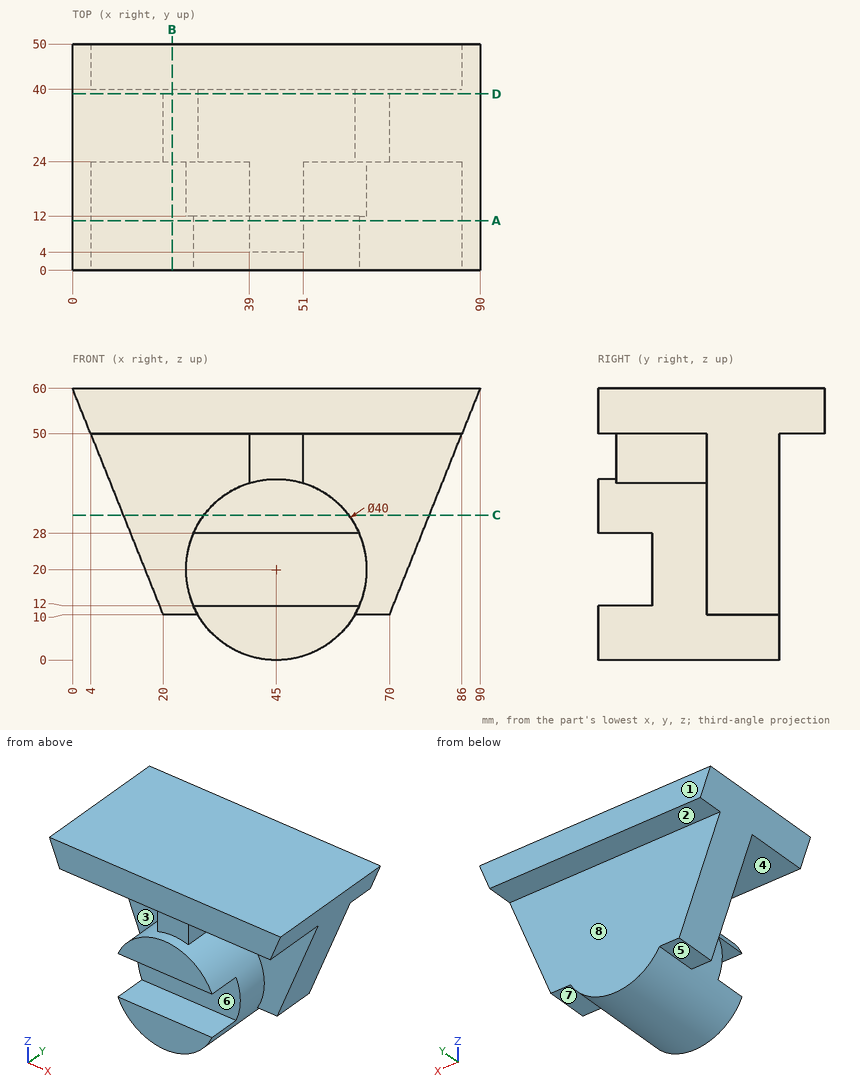
Design review of the part shown in the three views and the two pictorial views. Dimensions are in mm from the part's minimum x, y and z. A direction names the side the tool comes from. Give positions to 0.01 mm unless a question says otherwise; leave off trailing zeros. Write each loop counter-clockwise with the first axis right and the second up, starting at its lowest first coordinate (ties: lowest second). Pieces come first, ordered by that corner, then holes. Notation, with made-up numbers: M 70,36 L 95,36 A9 ccw 95,48 Z; hole C 74.25,-12 d3. An arc over 180 degrees is marked long. Answer in a Markdown table with one row per item.
Item 1: For line 1 along Y through (x, z) = (25, 23.5); line 2 along X through (y, z) = (16.5, 47.5); line 3 along Y through (x, z) = (54, 31.5), list the stretches that pass through material, from the lowest coordinate up.
Check sheet entries:
| item | result |
|---|---|
| line 1 | 24 to 40 |
| line 2 | 39 to 51 |
| line 3 | 0 to 40 |
Item 2: Draft analysis for pull direction Z (two halves, no side actions). For the marked faces 1, 2 and 3, state which applies: +Z half, -Z half, draft (parallel to the pull), parting line (faces both ways), or undercut.
Check sheet entries:
| item | result |
|---|---|
| face 1 | draft |
| face 2 | -Z half |
| face 3 | undercut |
Item 3: Add section B-B on x = 22. Give the boundary of the cut face in (y, z), plus the area to 3 significant figures.
Check sheet entries:
| item | result |
|---|---|
| outline | M 0,50 L 24,50 L 24,10 L 40,10 L 40,50 L 50,50 L 50,60 L 0,60 Z |
| area | 1,140 mm2 |
Item 4: Tool access review of the marked faces 4, 5, 6, 7 and 8: name each direction out of +Z, -Z, +X, -X, +Y, -Y from which nothing blocks a thin tool from reaching the whole face with its end or side.
Check sheet entries:
| item | result |
|---|---|
| face 4 | -Y |
| face 5 | -Z, -X, +Y, -Y |
| face 6 | +X, -X, -Y |
| face 7 | -Z, +X, +Y, -Y |
| face 8 | -Z, +X, -X, +Y |
Item 5: Add section A-A on y = 11. Give the boundary of the cut face in (x, z).
Check sheet entries:
| item | result |
|---|---|
| outline | M 0,60 L 4,50 L 39,50 L 39,39.08 A20 ccw 26.67,28 L 63.33,28 A20 ccw 51,39.08 L 51,50 L 86,50 L 90,60 Z; M 26.67,12 A20 ccw 63.33,12 Z |
Item 6: Add section C-C on z = 32. Give the boundary of the cut face in (x, y), plus the area to 3 significant figures.
Check sheet entries:
| item | result |
|---|---|
| outline | M 11.2,24 L 29,24 L 29,0 L 61,0 L 61,24 L 78.8,24 L 78.8,40 L 11.2,40 Z |
| area | 1,850 mm2 |
Item 7: Add section D-D on y = 39. Give the boundary of the cut face in (x, z).
Check sheet entries:
| item | result |
|---|---|
| outline | M 0,60 L 20,10 L 27.68,10 A20 ccw 62.32,10 L 70,10 L 90,60 Z |
Item 8: For P1, Ø1.5, axis at y = 13.5, z = 42, coming from the -X side; P2, Ø12, axis at y = 18.5, z = 34.5, coming from the -X side; P3, Ø2.5, axis at x = 25, y = 29.5, coming from the -Z side; P4, Ø1.5, axis at x = 79, z = 30, coming from the +Y side, all flat-tipped, find the tip position at first contact; note any pin that passes through.
Check sheet entries:
| item | result |
|---|---|
| P1 | x = 39 |
| P2 | x = 9.24 |
| P3 | z = 10 |
| P4 | through |
